Answer from the drawing. Dimensions are ordinates in mm from the lowest x, y and z of the part. Give positions to 0.01 mm unless a question says otherwise; leave off trailing zeros. Write each loop counter-clockwise with the first axis right and the second up, starting at its lowest first coordinate (ties: lowest second). Pieces come first, ordered by that corner, then holes. Notation, with made-up numbers: M -3,42.5 L 53,42.5 A7 ccw 53,50.5 Z; hole C 61.5,-15 d5. An arc over 180 degrees is marked long. Put each result on its own line as item: value.
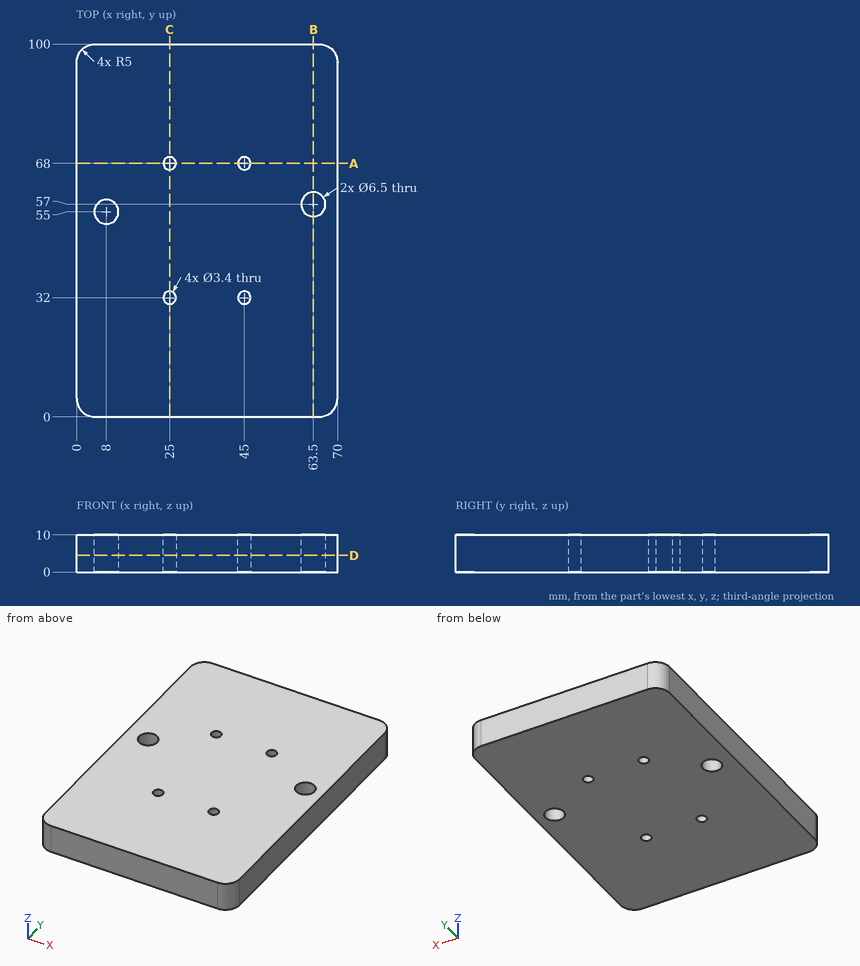
(1) Given pin 1 Ø4 at (x, y) = (8, 55) entering from -Z; pin 2 Ø4 at (x, z) = (45.5, 3.5) entering from -Y, each flat-ended and moving along its own axis, determine where each tip first touches the part or whether it passes through.
Result:
pin 1: passes through
pin 2: stops at y = 0
(2) Straight lines are drawn through the part: line 1 along X through (y, z) = (68, 3.75); line 2 along X through (y, z) = (68.5, 2); line 3 along Y through (x, z) = (24, 1). For each, find the intervals that lie inside material, in ascending order. Write a range as from..to.
Result:
line 1: x = 0..23.3, 26.7..43.3, 46.7..70
line 2: x = 0..23.38, 26.62..43.38, 46.62..70
line 3: y = 0..30.63, 33.37..66.63, 69.37..100
(3) Section A-A on y = 68 is taken. Determine the outline of the cut face in (x, z).
Result:
outline: M 0,0 L 23.3,0 L 23.3,10 L 0,10 Z; M 26.7,0 L 43.3,0 L 43.3,10 L 26.7,10 Z; M 46.7,0 L 70,0 L 70,10 L 46.7,10 Z
(4) Section B-B on x = 63.5 is taken. Determine the outline of the cut face in (y, z).
Result:
outline: M 0,0 L 53.75,0 L 53.75,10 L 0,10 Z; M 60.25,0 L 100,0 L 100,10 L 60.25,10 Z
(5) Section C-C on x = 25 is taken. Determine the outline of the cut face in (y, z).
Result:
outline: M 0,0 L 30.3,0 L 30.3,10 L 0,10 Z; M 33.7,0 L 66.3,0 L 66.3,10 L 33.7,10 Z; M 69.7,0 L 100,0 L 100,10 L 69.7,10 Z
(6) Section D-D on z = 4.5 is taken. Determine the outline of the cut face in (x, y).
Result:
outline: M 0,5 A5 ccw 5,0 L 65,0 A5 ccw 70,5 L 70,95 A5 ccw 65,100 L 5,100 A5 ccw 0,95 Z; hole C 8,55 d6.5; hole C 25,32 d3.4; hole C 25,68 d3.4; hole C 45,32 d3.4; hole C 45,68 d3.4; hole C 63.5,57 d6.5
